Check sheet for the modelled part. Datum: model origin and axes. Units: mm. A direction names the side the tool comes from. Coordinates: 2 decimals unless noted, no trailing zeros. Write each loop counter-clockwise with the first axis right and the second up, starting at its lowest first coordinate (ties: lowest second). Pieces come first, ordered by that corner, then holes. Notation, with made-up numbers: (-20, 47.25) - (8, 47.25) arc R25 ccw to (8, 82.25) - close; hole circle Ø5 at (-16.5, -33). An arc over 180 degrees is marked (long way). Use one line per item in the form item = value. Start each with the question number.
1. Scan lines: line 1 along X through (y, z) = (14, 19.5); line 2 along X through (y, z) = (35.55, -11.5); line 3 along X through (y, z) = (20, 15). Record each from-to range of solid material in increasing order.
2. Cross-section at D-D on z = -11.5. Record the boundary of the cut face in (x, y).
3. Go/stop test with flat-tipped pins: pin 1 Ø3 at (x, z) = (-8.5, 6.5) entering from -Y; pin 2 Ø6.5 at (x, z) = (-26.5, -11.5) entering from -Y. Record where each tip stops, or that it passes through.
4. Tool access check on faces 4 (the face through (0, 17, -20.5)), 5 (the face through (-10.94, 36.01, -12.04)). Record the directions out of +Z, -Z, +X, -X, +Y, -Y that give a thin tool (end or side, any length) a straight path to the whole face; none if there is none.
5. Cross-section at B-B on x = -26.5. Record the boundary of the cut face in (y, z), then the cut area to 3 significant figures.
6. Cross-section at C-C on y = 20. Record the boundary of the cut face in (x, z).
7. Cross-section at A-A on z = 19.5. Record the boundary of the cut face in (x, y).
8. Draft check along X on faces 1 (the face through (-1, 18, -22.5)), 2 (the face through (0, 17, 20.5)), 3 (the face through (38.5, 18, 0)). Enter one of: +X half, -X half, draft (parallel to the pull), parting line (faces both ways), or undercut.
```python
from build123d import *

# Parameters (mm, degrees)
SKETCH2_W            = 77
SKETCH2_H            = 45
BOSS_EXTRUDE1_DEPTH  = 37
SKETCH24_R           = 2
CUT_EXTRUDE13_DEPTH  = 58.943938423
SHELL2_T             = -2
SKETCH5_R            = 2.5
CUT_EXTRUDE1_DEPTH   = 58.943938423
LPATTERN1_COUNT      = 3
LPATTERN1_PITCH      = 9
LPATTERN2_COUNT      = 3
LPATTERN2_PITCH      = 9
LPATTERN2_COUNT_DIR2 = 3
LPATTERN2_PITCH_DIR2 = 9
SKETCH19_R           = 9
CUT_EXTRUDE11_DEPTH  = 2
FILLET1_R            = 2


with BuildPart() as part:
    # Sketch2 → Boss-Extrude1 (new body)
    with BuildSketch(Plane(origin=(0, 0, 0), x_dir=(1, 0, 0), z_dir=(0, 1, 0))):
        Rectangle(SKETCH2_W, SKETCH2_H)
    extrude(amount=BOSS_EXTRUDE1_DEPTH)

    # Sketch24 → Cut-Extrude13 (cut, through all)
    with BuildSketch(Plane.XZ):
        with Locations(Location((-35.5, 19.5, 0), (0, 0, 270))):
            Circle(SKETCH24_R)
        with Locations(Location((35.5, 19.5, 0), (0, 0, 90))):
            Circle(SKETCH24_R)
        with Locations(Location((35.5, -19.5, 0), (0, 0, 270))):
            Circle(SKETCH24_R)
        with Locations(Location((-35.5, -19.5, 0), (0, 0, 90))):
            Circle(SKETCH24_R)
    extrude(amount=-CUT_EXTRUDE13_DEPTH, mode=Mode.SUBTRACT)

    # Shell2
    shell2_openings = [part.faces().sort_by_distance(p)[0] for p in [
        (0, 0, 0),
    ]]
    offset(amount=SHELL2_T, openings=shell2_openings)

    # Sketch5 → Cut-Extrude1 (cut, through all)
    with BuildSketch(Plane(origin=(0, 37, 0), x_dir=(1, 0, 0), z_dir=(0, 1, 0))):
        with Locations(Location((-26.5, 11.5, 0), (0, 0, 270))):
            Circle(SKETCH5_R)
    cut_extrude1 = extrude(amount=-CUT_EXTRUDE1_DEPTH, mode=Mode.SUBTRACT)

    # LPattern1: Cut-Extrude1 ×3
    with Locations(*[(i * LPATTERN1_PITCH, 0, 0) for i in range(1, LPATTERN1_COUNT)]):
        add(cut_extrude1, mode=Mode.SUBTRACT)

    # LPattern2: Cut-Extrude1 3 × 3, 2 skipped
    with Locations(*[(j * LPATTERN2_PITCH_DIR2, 0, i * LPATTERN2_PITCH) for i in range(LPATTERN2_COUNT) for j in range(LPATTERN2_COUNT_DIR2) if (i, j) not in ((0, 0), (1, 0), (1, 2))]):
        add(cut_extrude1, mode=Mode.SUBTRACT)

    # Sketch19 → Cut-Extrude11 (cut)
    with BuildSketch(Plane(origin=(0, 37, 0), x_dir=(1, 0, 0), z_dir=(0, 1, 0))):
        with Locations(Location((23.5, 0, 0), (0, 0, 270))):
            Circle(SKETCH19_R)
    extrude(amount=-CUT_EXTRUDE11_DEPTH, mode=Mode.SUBTRACT)

    # Fillet1
    fillet1_edges = [part.edges().sort_by_distance(p)[0] for p in [
        (38.5, 18.5, 22.5),
        (-38.5, 18.5, 22.5),
        (-38.5, 18.5, -22.5),
        (38.5, 18.5, -22.5),
    ]]
    fillet(fillet1_edges, radius=FILLET1_R)


solid = part.part
```
Final values:
q1.line_1 = -38.5 to -37.5, -33.5 to -31.5, 31.5 to 33.5, 37.5 to 38.5
q1.line_2 = -38.5 to -29, -24 to -20, -15 to -11, -6 to 38.5
q1.line_3 = -38.5 to -36.5, 36.5 to 38.5
q2.outline = (-38.5, 0) - (-36.5, 0) - (-36.5, 35) - (-29, 35) - (-29, 37) - (-38.5, 37) - close; (-24, 35) - (-20, 35) - (-20, 37) - (-24, 37) - close; (-15, 35) - (-11, 35) - (-11, 37) - (-15, 37) - close; (-6, 35) - (36.5, 35) - (36.5, 0) - (38.5, 0) - (38.5, 37) - (-6, 37) - close
q3.pin_1 = through
q3.pin_2 = 35
q4.face_4 = -Y
q4.face_5 = +Y, -Y
q5.outline = (0, -22.5) - (37, -22.5) - (37, -14) - (35, -14) - (35, -20.5) - (0, -20.5) - close; (0, 20.5) - (35, 20.5) - (35, 9) - (37, 9) - (37, 22.5) - (0, 22.5) - close; (35, -9) - (37, -9) - (37, 4) - (35, 4) - close
q5.area = 210 mm²
q6.outline = (-38.5, -20.5) arc R2 ccw to (-36.5, -22.5) - (36.5, -22.5) arc R2 ccw to (38.5, -20.5) - (38.5, 20.5) arc R2 ccw to (36.5, 22.5) - (-36.5, 22.5) arc R2 ccw to (-38.5, 20.5) - close; hole circle Ø4 at (-35.5, -19.5); hole circle Ø4 at (-35.5, 19.5); hole (-36.5, -15.63) arc R4 cw to (-31.63, -20.5) - (31.63, -20.5) arc R4 cw to (36.5, -15.63) - (36.5, 15.63) arc R4 cw to (31.63, 20.5) - (-31.63, 20.5) arc R4 cw to (-36.5, 15.63) - close; hole circle Ø4 at (35.5, -19.5); hole circle Ø4 at (35.5, 19.5)
q7.outline = (-38.5, 0) - (-37.5, 0) - (-37.5, 37) - (-38.5, 37) - close; (-33.5, 0) - (-31.5, 0) - (-31.5, 35) - (31.5, 35) - (31.5, 0) - (33.5, 0) - (33.5, 37) - (-33.5, 37) - close; (37.5, 0) - (38.5, 0) - (38.5, 37) - (37.5, 37) - close
q8.face_1 = draft
q8.face_2 = undercut
q8.face_3 = +X half
